Can you work these out from the model? Positions are in its coordinate system, mm. A direction names the side the tool comes from. Give positions to 0.01 mm unless a question says otherwise; leave off trailing zeros. Order: outer loops, then holes, each group sorted by start corner. A loop starts at its lowest first (then second) coordinate and runs counter-clockwise, first axis right, second up. Notation, with made-up numbers: (65.25, -25) - (72.25, -25) arc R31 ccw to (72.25, 12) - close; hole circle Ø6 at (23, 11.25). An arc over 180 degrees is marked (long way). Use one line per item in the form item = value. Start each with the question number.
1) Suppose I cut it at C-C, the plane x = 57.5. Write out the boundary of the cut face in (y, z), and give its area (3 significant figures).
2) Which directions (+Z, -Z, +X, -X, +Y, -Y) give clear straight access to the entire face, cutting with the end or side of a thin tool? Please do faces 1 (the cylindrical face through (0, 44, 78)), 2 (the cylindrical face through (60.273, -11.645, 76.26)).
3) Please list where these lines run through material, in increasing order: probe 1 along Y at (x, z) = (-57, 76.85); probe 2 along X at (y, z) = (40, 75.9); probe 3 along X at (y, z) = (-44, 76.1).
4) Suppose I cut it at B-B, the plane y = -20.5. Write out the boundary of the cut face in (x, z), and give its area (3 significant figures).
5) Suppose I cut it at A-A, the plane x = 0. State how many separate pieces and enclosed holes the cut face has, and give its area (3 significant figures).
6) We'd pull the mould along X, two halves only. Please class faces 3 (the flat face through (0, 64, 75.5)), 4 (the flat face through (-29, -50, 78.524)), 5 (the cylindrical face through (-23.955, -49.585, 77.751)): released by +X, released by -X, zero draft, split by the parting line, or undercut.
7) Suppose I cut it at D-D, the plane y = -40. Write out the boundary of the cut face in (x, z).
8) For pin 1 (11 mm diameter, centred on x = 0, y = -40, fed in from -Z); pin 2 (1 mm diameter, centred on x = -14.5, z = 76, fed in from +Y); pin 3 (8 mm diameter, centred on x = 35.507, y = -20.5, fed in from +Z); pin 4 (5 mm diameter, centred on x = 28.5, y = -48.5, fed in from -Z), each with a flat end and sliding along its axis, tell me the tip position at first contact or that it passes through.
Autodesk Inventor part; units mm, degrees
ref_plane "Work Plane1" through (0, 0, 55) normal (0, 0, 1) x (1, 0, 0)
ref_plane "Work Plane4" through (0, 68, 0) normal (0, 1, 0) x (-1, 0, 0)
ref_plane "YZ Plane" through (0, 0, 0) normal (1, 0, 0) x (0, 1, 0)
sketch "Sketch1" plane through (0, 0, 0) normal (0, 0, 1) x (1, 0, 0)
  circle A0 centre (0, 0) radius 68
  dimension "d1" = 136
extrude "Extrusion1" add sketch "Sketch1" along normal blind 80
shell "Shell1" thickness 3 removed faces 1 at (13.6377, 7.7647, 0)
sketch "Sketch2" plane through (0, 0, 80) normal (0, 0, 1) x (1, 0, 0)
  circle A0 centre (0, 0) radius 32
  dimension "d5" = 64
extrude "Extrusion2" cut sketch "Sketch2" against normal up to surface (3 mm away)
sketch "Sketch3" plane through (0, 0, 77) normal (0, 0, -1) x (-1, 0, 0)
  circle A0 centre (0, 0) radius 32
  circle A1 centre (0, 0) radius 65
  circle A2 centre (0, -40) radius 4.8
  line L0 (0, 0) -> (0, -56.282) construction
  line L1 (0, 0) -> (-47.9956, 27.7103) construction
  line L2 (0, 0) -> (60.1339, 34.7183) construction
  circle A3 centre (-34.641, 20) radius 4.8
  circle A4 centre (34.641, 20) radius 4.8
  dimension "d8" = 9.6
  dimension "d9" = 40
  dimension "d10" = 120
  dimension "d11" = 120
  dimension "d12" = 9.6
  dimension "d13" = 9.6
  dimension "d14" = 40
  dimension "d15" = 40
extrude "Extrusion3" cut sketch "Sketch3" against normal blind 1.524 contours A2 | A3 | A4
ref_plane "Work Plane1" through (0, 0, 55) normal (0, 0, 1) x (1, 0, 0)
sketch "Sketch4" plane through (0, 0, 55) normal (0, 0, 1) x (1, 0, 0)
  circle A0 centre (0, 0) radius 68
  circle A1 centre (0, 0) radius 68
  line L0 (0, 68) -> (56.3915, 68)
  line L1 (56.3915, 68) -> (56.3915, 38)
  line L2 (56.3915, 38) -> (0, 38)
  line L3 (0, 38) -> (0, 68)
  dimension "d24" = 30
extrude "Extrusion4" add sketch "Sketch4" against normal blind 25 contours A0 L0 L1
sketch "Sketch6" plane through (56.3915, 38, 55) normal (1, 0, 0) x (0, 0, -1)
  line L0 (0, 0) -> (0, 30)
  line L1 (25, 0) -> (0, 0)
  line L2 (25, 30) -> (25, 0)
  line L3 (0, 30) -> (25, 30)
  line L4 (22, 27) -> (22, 3)
  line L5 (22, 3) -> (3, 3)
  line L6 (3, 3) -> (3, 27)
  line L7 (3, 27) -> (22, 27)
  point P0 (55, -38)
  dimension "d27" = 3
extrude "Extrusion5" cut sketch "Sketch6" against normal blind 56.391 contours L4 L5 L6 L7
ref_plane "Work Plane4" through (0, 68, 0) normal (0, 1, 0) x (-1, 0, 0)
sketch "Sketch9" plane through (56.3915, 38, 55) normal (1, 0, 0) x (0, 0, -1)
  line L0 (3, 3) -> (3, 27)
  line L1 (3, 27) -> (22, 27)
  line L2 (22, 27) -> (22, 3)
  line L3 (22, 3) -> (3, 3)
  line L4 (0, 0) -> (0, 30)
  line L5 (25, 0) -> (0, 0)
  line L6 (25, 30) -> (25, 0)
  line L7 (0, 30) -> (25, 30)
  point P0 (55, -38)
sketch "Sketch10" plane through (0, 68, 0) normal (0, 1, 0) x (-1, 0, 0)
  circle A0 centre (-56.3915, 0) radius 55 construction
  line L0 (-127.7058, 55) -> (100.6176, 55)
  line L1 (-56.3915, 55) -> (0, 55)
  line L2 (0, 0) -> (-96.3915, 0) construction
  arc A1 (-56.3915, 55) -> (-111.3915, 0) centre (-56.3915, 0) ccw
sweep "Sweep2" add profiles "Sketch9" path "Sketch10" path curves A1
sketch "Sketch11" plane through (0, 0, 77) normal (0, 0, -1) x (-1, 0, 0)
  circle A0 centre (-34.641, 20) radius 4.8
  circle A1 centre (34.641, 20) radius 4.8
  circle A2 centre (0, -40) radius 4.8
  circle A3 centre (0, 0) radius 32
  circle A4 centre (0, 0) radius 65
  circle A5 centre (-34.641, 20) radius 6.3
  circle A6 centre (34.641, 20) radius 6.3
  circle A7 centre (0, -40) radius 6.3
  circle A8 centre (0, 0) radius 33.5
  line L0 (-36.0415, 26.1424) -> (-7.4468, 32.6618)
  line L1 (-40.6607, 18.1416) -> (-32.0094, -9.8818)
  line L2 (36.0415, 26.1424) -> (7.4468, 32.6618)
  line L3 (40.6607, 18.1416) -> (32.0094, -9.8818)
  line L4 (4.6192, -44.284) -> (24.5626, -22.78)
  line L5 (-4.6192, -44.284) -> (-24.5626, -22.78)
  circle A9 centre (-34.641, 20) radius 7.8
  line L6 (-42.0939, 17.6992) -> (-34.7194, -6.1884)
  circle A10 centre (34.641, 20) radius 7.8
  circle A11 centre (0, -40) radius 7.8
  line L7 (-36.3749, 27.6048) -> (-12.0004, 33.1621)
  line L8 (36.3749, 27.6048) -> (12.0004, 33.1621)
  line L9 (42.0939, 17.6992) -> (34.7194, -6.1884)
  line L10 (5.7191, -45.304) -> (22.7191, -26.9737)
  line L11 (-5.7191, -45.304) -> (-22.7191, -26.9737)
  line L12 (-34.7194, -6.1884) -> (-33.2862, -5.746)
  line L13 (-22.7191, -26.9737) -> (-21.6192, -25.9537)
  line L14 (12.0004, 33.1621) -> (11.6669, 31.6997)
  line L15 (34.7194, -6.1884) -> (33.2862, -5.746)
  line L16 (22.7191, -26.9737) -> (21.6192, -25.9537)
  line L17 (-12.0004, 33.1621) -> (-11.6669, 31.6997)
  dimension "d39" = 1.5
  dimension "d40" = 1.5
  dimension "d41" = 1.5
  dimension "d42" = 1.5
  dimension "d43" = 1.5
  dimension "d44" = 1.5
  dimension "d45" = 1.5
  dimension "d46" = 25
  dimension "d47" = 25
  dimension "d48" = 25
  dimension "d49" = 25
  dimension "d50" = 25
  dimension "d51" = 25
extrude "Extrusion6" add sketch "Sketch11" along normal blind 1.5 contours A5 L1 A9 L0 | A9 L7 L17 L0 | L1 L12 L6 A9 | L14 L8 A10 L2 | L5 A11 L11 L13 | A10 L3 A6 L2 | L5 A7 L4 A11 | A10 L9 L15 L3 | L16 L10 A11 L4
sketch "Sketch14" plane through (0, 0, 80) normal (0, 0, 1) x (1, 0, 0)
  circle A0 centre (0, 0) radius 32
  line L0 (0, 0) -> (0, 28.9416) construction
  circle A1 centre (0, 41) radius 3
  line L1 (0, 0) -> (-25.0642, -14.4708) construction
  line L2 (0, 0) -> (25.0642, -14.4708) construction
  point P0 (-35.507, -20.5)
  point P1 (-35.507, -20.5)
  point P2 (35.507, -20.5)
  point P3 (35.507, -20.5)
  dimension "d98" = 6
  dimension "d99" = 41
  dimension "d102" = 360
hole "Hole1" at (0, 41, 80) at (-35.507, -20.5, 80) at (35.507, -20.5, 80) direction (0, 0, -1) diameter 6 end through all
sketch "Sketch16" plane through (0, 0, 0) normal (0, 0, -1) x (-1, 0, 0)
  circle A0 centre (0, 0) radius 68
  line L0 (-147.0847, -150.1925) -> (110.1745, -150.1925)
  line L1 (110.1745, -150.1925) -> (110.1745, 168.3901)
  line L2 (110.1745, 168.3901) -> (-147.0847, 168.3901)
  line L3 (-147.0847, 168.3901) -> (-147.0847, -150.1925)
extrude "Extrusion9" cut sketch "Sketch16" against normal up to surface (75.5 mm away) contours A0 | L3 L2 L1 L0
sketch "Sketch17" plane through (0, 0, 75.5) normal (0, 0, -1) x (-1, 0, 0)
  circle A0 centre (0, 0) radius 65
  circle A1 centre (0, 0) radius 68
extrude "Extrusion10" cut sketch "Sketch17" against normal up to surface (1.5 mm away)
sketch "Sketch18" plane through (0, 0, 77) normal (0, 0, -1) x (-1, 0, 0)
  circle A0 centre (0, 0) radius 68
  circle A1 centre (0, 0) radius 71
  line L0 (0, 0) -> (-80.0299, 0) construction
  circle A2 centre (-57.5, 0) radius 4.8
  circle A3 centre (0, 0) radius 65
  circle A4 centre (-57.5, 0) radius 6.3
  circle A5 centre (-52.744, -15.5907) radius 10
  circle A6 centre (-52.744, 15.5907) radius 10
  circle A7 centre (-12.87, -53.473) radius 10
  circle A8 centre (-28.75, -49.7965) radius 6.3
  circle A9 centre (-28.75, -49.7965) radius 4.8
  circle A10 centre (-39.874, -37.8823) radius 10
  circle A11 centre (39.874, -37.8823) radius 10
  circle A12 centre (28.75, -49.7965) radius 6.3
  circle A13 centre (28.75, -49.7965) radius 4.8
  circle A14 centre (12.87, -53.473) radius 10
  circle A15 centre (52.744, 15.5907) radius 10
  circle A16 centre (57.5, 0) radius 6.3
  circle A17 centre (57.5, 0) radius 4.8
  circle A18 centre (52.744, -15.5907) radius 10
  circle A19 centre (12.87, 53.473) radius 10
  circle A20 centre (28.75, 49.7965) radius 6.3
  circle A21 centre (28.75, 49.7965) radius 4.8
  circle A22 centre (39.874, 37.8823) radius 10
  circle A23 centre (-39.874, 37.8823) radius 10
  circle A24 centre (-28.75, 49.7965) radius 6.3
  circle A25 centre (-28.75, 49.7965) radius 4.8
  circle A26 centre (-12.87, 53.473) radius 10
  circle A27 centre (-52.744, -15.5907) radius 8.5
  circle A28 centre (-39.874, -37.8823) radius 8.5
  circle A29 centre (0, 0) radius 63.5
  line L1 (-33.0494, -45.1916) -> (-34.0731, -44.0952)
  line L2 (-55.6618, -6.0259) -> (-55.2241, -7.4606)
  circle A30 centre (-12.87, -53.473) radius 8.5
  circle A31 centre (12.87, -53.473) radius 8.5
  line L3 (-22.6123, -51.2175) -> (-21.151, -51.5558)
  line L4 (22.6123, -51.2175) -> (21.151, -51.5558)
  circle A32 centre (39.874, -37.8823) radius 8.5
  circle A33 centre (52.744, -15.5907) radius 8.5
  line L5 (33.0494, -45.1916) -> (34.0731, -44.0952)
  line L6 (55.6618, -6.0259) -> (55.2241, -7.4606)
  circle A34 centre (52.744, 15.5907) radius 8.5
  circle A35 centre (39.874, 37.8823) radius 8.5
  line L7 (55.6618, 6.0259) -> (55.2241, 7.4606)
  line L8 (33.0494, 45.1916) -> (34.0731, 44.0952)
  circle A36 centre (12.87, 53.473) radius 8.5
  circle A37 centre (-12.87, 53.473) radius 8.5
  line L9 (22.6123, 51.2175) -> (21.151, 51.5558)
  line L10 (-22.6123, 51.2175) -> (-21.151, 51.5558)
  circle A38 centre (-39.874, 37.8823) radius 8.5
  circle A39 centre (-52.744, 15.5907) radius 8.5
  line L11 (-33.0494, 45.1916) -> (-34.0731, 44.0952)
  line L12 (-55.6618, 6.0259) -> (-55.2241, 7.4606)
  point P0 (22.6123, -51.2175)
  point P1 (14.859, -61.737)
  point P2 (-14.859, -61.737)
  point P3 (-22.6123, -51.2175)
  point P4 (-15.2101, -63.1954)
  point P5 (15.2101, -63.1954)
  point P6 (55.6618, -6.0259)
  point P7 (60.8953, -18.0002)
  point P8 (46.0363, -43.7368)
  point P9 (33.0494, -45.1916)
  point P10 (47.1238, -44.77)
  point P11 (62.3338, -18.4254)
  point P12 (33.0494, 45.1916)
  point P13 (46.0363, 43.7368)
  point P14 (60.8953, 18.0002)
  point P15 (55.6618, 6.0259)
  point P16 (62.3338, 18.4254)
  point P17 (47.1238, 44.77)
  point P18 (-22.6123, 51.2175)
  point P19 (-14.859, 61.737)
  point P20 (14.859, 61.737)
  point P21 (15.2101, 63.1954)
  point P22 (-15.2101, 63.1954)
  point P23 (-55.6618, 6.0259)
  point P24 (-60.8953, 18.0002)
  point P25 (-46.0363, 43.7368)
  point P26 (-33.0494, 45.1916)
  point P27 (-47.1238, 44.77)
  point P28 (-62.3338, 18.4254)
  point P29 (-60.8953, -18.0002)
  point P30 (-62.3338, -18.4254)
  point P31 (-47.1238, -44.77)
  point P32 (-46.0363, -43.7368)
  dimension "d120" = 20
  dimension "d126" = 1.5
  dimension "d127" = 1.5
  dimension "d115" = 142
  dimension "d116" = 9.6
  dimension "d117" = 130
  dimension "d118" = 57.5
  dimension "d119" = 1.5
  dimension "d121" = 20
  dimension "d124" = 360
  dimension "d130" = 360
extrude "Extrusion11" add sketch "Sketch18" along normal blind 1.5 contours A1 | A15 A29 A22 A3 | A15 A29 | A3 A11 A29 A18 | A18 A29 | A22 A29 | A11 A29 | A19 A29 A26 A3 | A19 A29 | A29 A35 L8 A22 | A15 L7 A34 A29 | A3 A7 A29 A14 | A14 A29 | A11 L5 A32 A29 | A18 A29 A33 L6 | A26 A29 | A19 L9 A36 A29 | A7 A29 | A29 A31 L4 A14 | A23 A29 A6 A3 | A23 A29 | A29 A37 L10 A26 | A3 A5 A29 A10 | A10 A29 | A7 L3 A30 A29 | A6 A29 | A23 L11 A38 A29 | A5 A29 | A29 A28 L1 A10 | A29 A39 L12 A6 | A5 L2 A27 A29 picked at (34.5421, 45.674) picked at (56.7995, 7.0624) picked at (34.5421, -45.6741) picked at (56.7995, -7.0624) picked at (22.201, 54.9051) picked at (22.201, -54.9051) picked at (-22.2838, 52.7514) picked at (-22.2838, -52.7514) picked at (-34.5421, 45.6741) picked at (-34.5421, -45.674) picked at (-56.826, 7.0773) picked at (-56.826, -7.0773)
sketch "Sketch20" plane through (0, 0, 77) normal (0, 0, 1) x (1, 0, 0)
  circle A0 centre (0, 0) radius 71
  circle A1 centre (0, 0) radius 68
  circle A2 centre (0, 0) radius 68
extrude "Extrusion13" add sketch "Sketch20" along normal up to surface (3 mm away)
sketch "Sketch19" plane through (0, 0, 77) normal (0, 0, -1) x (-1, 0, 0)
  line L0 (0, 0) -> (-65.5735, 0) construction
  circle A0 centre (-57.5, 0) radius 4.8
  circle A1 centre (-28.75, -49.7965) radius 4.8
  circle A2 centre (28.75, -49.7965) radius 4.8
  circle A3 centre (57.5, 0) radius 4.8
  circle A4 centre (28.75, 49.7965) radius 4.8
  circle A5 centre (-28.75, 49.7965) radius 4.8
  dimension "d134" = 9.6
  dimension "d135" = 57.5
  dimension "d138" = 360
extrude "Extrusion12" cut sketch "Sketch19" against normal blind 1.524
equation "\"d11\" = d10"
equation "\"d12\" = d8"
equation "\"d13\" = d8"
equation "\"d40\" = d39"
equation "\"d41\" = d39"
equation "\"d42\" = d39"
equation "\"d44\" = d43"
equation "\"d45\" = d41"
equation "\"d47\" = d46"
equation "\"d48\" = d47"
equation "\"d49\" = d48"
equation "\"d50\" = d49"
equation "\"d51\" = d50"
equation "\"d127\" = d126"
equation "\"d121\" = d120"
properties part number "Top Lid"
Result sheet:
q1.outline = (-41.65, 75.5) - (-36.3, 75.5) - (-36.3, 77) - (-30.31, 77) - (-30.31, 75.5) - (-26.94, 75.5) - (-26.94, 77) - (-8.55, 77) - (-8.55, 75.5) - (-6.79, 75.5) - (-6.79, 77) - (-4.8, 77) - (-4.8, 78.52) - (4.8, 78.52) - (4.8, 77) - (6.79, 77) - (6.79, 75.5) - (8.55, 75.5) - (8.55, 77) - (26.94, 77) - (26.94, 75.5) - (30.31, 75.5) - (30.31, 77) - (36.3, 77) - (36.3, 75.5) - (41.65, 75.5) - (41.65, 80) - (-41.65, 80) - close
q1.area = 267 mm²
q2.face_1 = +Z, -Z
q2.face_2 = -Z
q3.probe_1 = -42.33 to -37.08, -31.24 to -27.99, -8.23 to -6.54, 6.54 to 8.23, 27.99 to 31.24, 37.08 to 42.33
q3.probe_2 = -58.66 to -54.99, -51.23 to -49.32, 49.32 to 51.23, 54.99 to 58.66
q3.probe_3 = -55.72 to -51.85, -47.84 to -45.78, -6.93 to -4.88, 4.88 to 6.93, 45.78 to 47.84, 51.85 to 55.72
q4.outline = (-67.98, 75.5) - (-64.84, 75.5) - (-64.84, 77) - (-61.68, 77) - (-61.68, 75.5) - (-60.1, 75.5) - (-60.1, 77) - (-38.51, 77) - (-38.51, 80) - (-67.98, 80) - close; (-32.51, 77) - (-24.57, 77) - (-24.57, 80) - (-32.51, 80) - close; (24.57, 77) - (32.51, 77) - (32.51, 80) - (24.57, 80) - close; (38.51, 77) - (60.1, 77) - (60.1, 75.5) - (61.68, 75.5) - (61.68, 77) - (64.84, 77) - (64.84, 75.5) - (67.98, 75.5) - (67.98, 80) - (38.51, 80) - close
q4.area = 239 mm²
q5.separate_pieces = 3
q5.enclosed_holes = 0
q5.area = 217 mm²
q6.face_3 = zero draft
q6.face_4 = undercut
q6.face_5 = undercut
q7.outline = (-58.66, 75.5) - (-54.99, 75.5) - (-54.99, 77) - (-51.23, 77) - (-51.23, 75.5) - (-49.32, 75.5) - (-49.32, 77) - (-10.64, 77) - (-10.64, 75.5) - (-8.59, 75.5) - (-8.59, 77) - (-4.8, 77) - (-4.8, 78.52) - (4.8, 78.52) - (4.8, 77) - (8.59, 77) - (8.59, 75.5) - (10.64, 75.5) - (10.64, 77) - (49.32, 77) - (49.32, 75.5) - (51.23, 75.5) - (51.23, 77) - (54.99, 77) - (54.99, 75.5) - (58.66, 75.5) - (58.66, 80) - (-58.66, 80) - close
q8.pin_1 = 77
q8.pin_2 = 69.61
q8.pin_3 = 80
q8.pin_4 = 78.52
